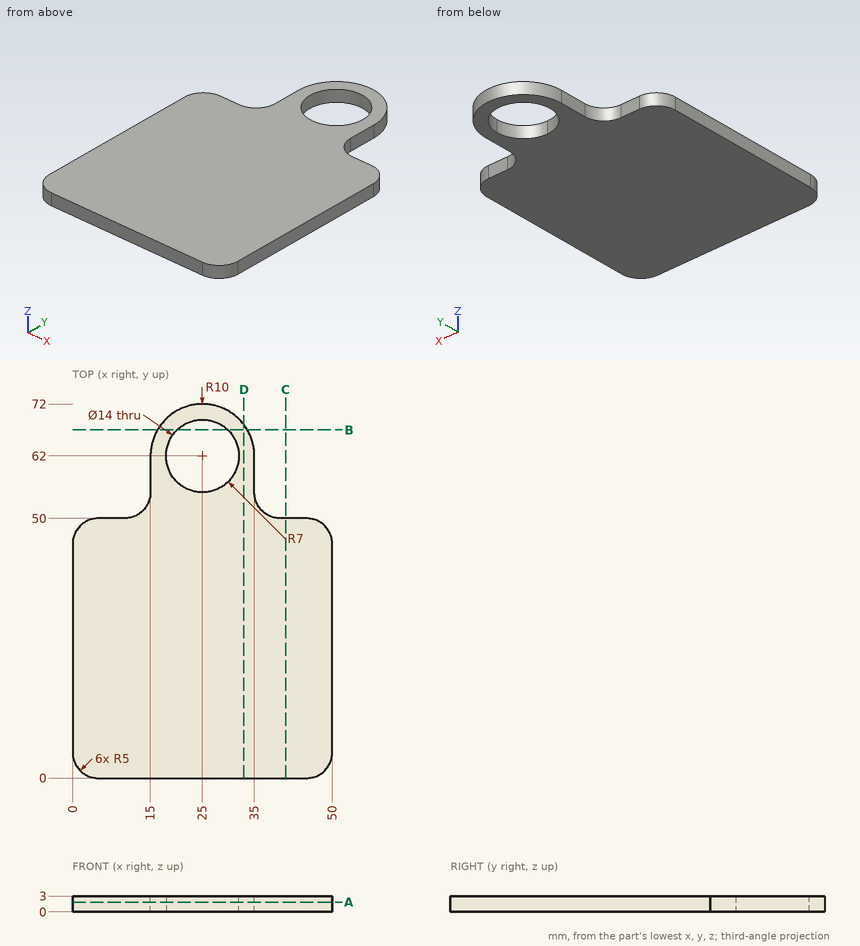
Verification items for this drawing (mm, ordinates from the low corner). Give positions to 0.01 mm unless a question says otherwise; leave off trailing zeros. Loops run counter-clockwise (first coordinate to the right, second up) from the corner with the lowest first, then second, coordinate; pieces in that order, holes last. Notation, with made-up numbers: (-10.75, 55) - (2.25, 55) arc R24 ccw to (2.25, 78) - close; hole circle Ø10 at (30, 45). An arc over 180 degrees is marked (long way). Write item = value, one per line. Start each with the question number.
Q1. Cross-section at D-D, the plane x = 33. Enter the section's corners in (y, z), and give its area (3 significant figures).
Q2. Cross-section at A-A, the plane z = 1.85. Enter the section's corners in (x, y).
Q3. Cross-section at C-C, the plane x = 41. Enter the section's corners in (y, z), and give its area (3 significant figures).
Q4. Thickness scan on line 1 (Y direction, x = 9.5, z = 2.95); line 2 (Y direction, x = 29, z = 2.2); line 3 (X direction, y = 67, z = 2.3). Record the ranges inside material, lowest first.
Q5. Cross-section at B-B, the plane y = 67. Enter the section's corners in (x, z).
Q6. Depth check by flat-ended pin: P1, Ø12.5, axis at x = 25, y = 62, coming from the +Z side; P2, Ø1.5, axis at x = 43.5, z = 2, coming from the +Y side; P3, Ø1, axis at y = 64, z = 2, coming from the -X side; P4, Ø1.5, axis at y = 57, z = 1, coming from the +X side. Enter the tip coordinate at first touch or a pass-through.
Answer key:
q1.outline = (0, 0) - (68, 0) - (68, 3) - (0, 3) - close
q1.area = 204 mm^2
q2.outline = (0, 5) arc R5 ccw to (5, 0) - (45, 0) arc R5 ccw to (50, 5) - (50, 45) arc R5 ccw to (45, 50) - (40, 50) arc R5 cw to (35, 55) - (35, 62) arc R10 ccw to (15, 62) - (15, 55) arc R5 cw to (10, 50) - (5, 50) arc R5 ccw to (0, 45) - close; hole (25, 55) arc R7 ccw to (32, 62) arc R7 ccw (long way) to start
q3.outline = (0, 0) - (50, 0) - (50, 3) - (0, 3) - close
q3.area = 150 mm^2
q4.line_1 = 0 to 50
q4.line_2 = 0 to 56.26, 67.74 to 71.17
q4.line_3 = 16.34 to 20.1, 29.9 to 33.66
q5.outline = (16.34, 0) - (20.1, 0) - (20.1, 3) - (16.34, 3) - close; (29.9, 0) - (33.66, 0) - (33.66, 3) - (29.9, 3) - close
q6.P1 = through
q6.P2 = 50
q6.P3 = 15.11
q6.P4 = 35
